The listing builds one solid part. Answer for the finished solid, in the listing's coordinates (mm). A direction names the side the tool comes from. Coordinates: 2 decimals unless noted, no trailing zeros. Write each loop counter-clockwise with the first axis right and the second up, starting at its lowest first coordinate (ties: lowest second). Pieces come first, ordered by that corner, then holes.
(1) The part is cut by section D-D on y = 13.5. Determine the outline of the cut face in (x, z), plus the area to 3 significant figures.
(2) Given P1, Ø2, axis at x = 39.5, y = 8, coming from the -Z side; P2, Ø4, axis at y = 19.5, z = 50, coming from the +X side; P3, Ø5, axis at x = 16.5, z = 44, coming from the +Y side, each flat-ended and moving along its own axis, determine where each tip first touches the part or whether it passes through.
(3) Which of the six approach directions +Z, -Z, +X, -X, +Y, -Y give full straight-line access (tool end or side, diameter ignored) to faces 1 (the flat face through (1, 21.5, 17)), 2 (the flat face through (29, 3, 38)), 3 (the flat face through (33, 2, 0))?
(4) The part is cut by section A-A on z = 50. Determine the outline of the cut face in (x, y), plus the area to 3 significant figures.
(5) The part is cut by section B-B on y = 18.5. Determine the outline of the cut face in (x, z).
(6) Straight lines are drawn through the part: line 1 (X direction, y = 15.25, z = 21); line 2 (Y direction, x = 0.6, z = 50); line 3 (Y direction, x = 33.5, z = 10.5). For each, find the intervals that lie inside material, in ascending order.
(7) For a pull along Y with two mould halves and no side action, classify faces 4 (the cylindrical face through (1.48, 21.61, 51.34)), 5 (the flat face through (62, 13, 40)), 6 (the flat face through (58, 25, 45)) as +Y half, -Y half, draft (parallel to the pull), parting line (faces both ways), or undercut.
(8) The part is cut by section C-C on z = 34.5. Determine the outline of the cut face in (x, y), plus the area to 3 significant figures.
Autodesk Inventor part; units mm, degrees
ref_plane "YZ Plane" through (0, 0, 0) normal (1, 0, 0) x (0, 1, 0)
ref_plane "XZ Plane" through (0, 0, 0) normal (0, 1, 0) x (-1, 0, 0)
ref_plane "XY Plane" through (0, 0, 0) normal (0, 0, 1) x (1, 0, 0)
sketch "Sketch2" plane through (0, 0, 0) normal (0, 1, 0) x (-1, 0, 0)
  line L0 (0, 0) -> (-59, 0)
  line L1 (-59, 0) -> (-59, 78)
  line L2 (-59, 78) -> (0, 78)
  line L3 (0, 78) -> (0, 0)
  dimension "d0" = 59
  dimension "d1" = 78
extrude "Extrusion1" add sketch "Sketch2" along normal blind 25
shell "Shell1" thickness 3 removed faces 1 at (39.3333, 25, 52)
sketch "Sketch4" plane through (59, 0, 0) normal (0, 0, -1) x (-1, 0, 0)
  point P0 (59, 0)
sketch "Sketch5" plane through (3, 3, 3) normal (0, 0, 1) x (1, 0, 0)
  line L0 (0, 0) -> (0, 22)
  line L1 (0, 22) -> (53, 22)
  line L2 (0, 0) -> (53, 0)
  line L3 (53, 0) -> (53, 22)
  line L4 (53, 22) -> (0, 22)
  line L5 (0, 22) -> (0, 0)
  point P0 (-3, -3)
extrude "Extrusion3" cut sketch "Sketch5" against normal blind 10
sketch "Sketch6" plane through (0, 0, 0) normal (-1, 0, 0) x (0, 0, 1)
  line L0 (4.5, 21.5) -> (30.5, 21.5)
  line L1 (30.5, 21.5) -> (30.5, 17.5)
  line L2 (30.5, 17.5) -> (4.5, 17.5)
  line L3 (4.5, 17.5) -> (4.5, 21.5)
  line L4 (0, 0) -> (0, 25)
  line L5 (0, 0) -> (78, 0)
  dimension "d19" = 26
  dimension "d20" = 4
  dimension "d21" = 4.5
  dimension "d22" = 17.5
sketch "Sketch7" plane through (59, 0, 78) normal (1, 0, 0) x (0, 0, -1)
  line L0 (0, 0) -> (78, 0)
  line L1 (0, 25) -> (78, 25)
  line L2 (78, 25) -> (78, 0)
  line L3 (78, 0) -> (0, 0)
  line L4 (0, 0) -> (0, 25)
extrude "Extrusion5" add sketch "Sketch7" along normal blind 3
extrude "Extrusion6" cut sketch "Sketch6" against normal through all
sketch "Sketch8" plane through (0, 0, 0) normal (-1, 0, 0) x (0, 0, 1)
  circle A0 centre (50, 19.5) radius 2.5
  point P0 (0, 0)
  dimension "d29" = 5
extrude "Extrusion7" cut sketch "Sketch8" against normal through all
properties part number "arduino box v05"
Model answer:
1. outline: (0, 0) - (3, 0) - (3, 75) - (56, 75) - (56, 0) - (62, 0) - (62, 78) - (0, 78) - close
1. area: 861 mm2
2. P1: stops at z = 75
2. P2: passes through
2. P3: stops at y = 3
3. face 1: +X, -X
3. face 2: -Z, +Y
3. face 3: -Z, +X, -X, +Y, -Y
4. outline: (0, 0) - (62, 0) - (62, 17) - (56, 17) - (56, 3) - (3, 3) - (3, 17) - (0, 17) - close; (0, 22) - (3, 22) - (3, 25) - (0, 25) - close; (56, 22) - (62, 22) - (62, 25) - (56, 25) - close
4. area: 339 mm2
5. outline: (0, 0) - (3, 0) - (3, 4.5) - (0, 4.5) - close; (0, 30.5) - (3, 30.5) - (3, 47.71) - (0, 47.71) - close; (0, 52.29) - (3, 52.29) - (3, 75) - (56, 75) - (56, 52.29) - (62, 52.29) - (62, 78) - (0, 78) - close; (56, 0) - (62, 0) - (62, 4.5) - (56, 4.5) - close; (56, 30.5) - (62, 30.5) - (62, 47.71) - (56, 47.71) - close
6. line 1: x = 0 to 3, 56 to 62
6. line 2: y = 0 to 17, 22 to 25
6. line 3: y = 0 to 3
7. face 4: undercut
7. face 5: draft
7. face 6: +Y half
8. outline: (0, 0) - (62, 0) - (62, 25) - (56, 25) - (56, 3) - (3, 3) - (3, 25) - (0, 25) - close
8. area: 384 mm2
